Geometry: final body of the model. Coordinates: model frame, mm. Face numbers are marked on the shaded views. A direction names the side the tool comes from. Coordinates: 2 decimals unless noted, no trailing zeros. Write each loop counter-clockwise with the first axis right and the second up, starting at its lowest first coordinate (ties: lowest second). Pieces come first, ordered by that corner, then holes. Notation, with made-up numbers: M 68.25,5.5 L 87.25,5.5 A33 ccw 87.25,34.5 Z; hole C 78,62 d7. An arc over 180 degrees is marked long. Write item = value, one per line. Start each with the question number.
Item 1: First-contact query: pin 1 Ø10 at (x, z) = (-21.5, 1.5) entering from -Y; pin 2 Ø3 at (y, z) = (-2.5, -4) entering from +X; pin 3 Ø1.5 at (y, z) = (16.5, 2) entering from -X. Flat tips, straight axial feed; report the tip coordinate or a pass-through.
Item 2: Pull-direction query (X, two-part tool) for the marked faces 3, 4 and 5; classes: +X half, -X half, draft (parallel to the pull), parting line (faces both ways), or undercut.
Item 3: Section B-B on z = -39. Output: boundary loops of the cut face in (x, y).
Item 4: Section A-A on z = 25. Output: boundary loops of the cut face in (x, y).
Item 5: Reachability of the marked faces 1 and 2 from +Z, -Z, +X, -X, +Y, -Y: full face, straight path, thin tool, end or side. Return the list, or none.
Item 6: Ray query, L1, parallel to Y at x = 0, z = 20; L2, parallel to Z at x = -8.5, y = 2.5; L3, parallel to X at y = -14.5, z = 9.5. Return the intervals inside material, ascending. Write a range as [from, to].
Autodesk Inventor part; units mm, degrees
ref_plane "YZ Plane" through (0, 0, 0) normal (1, 0, 0) x (0, 1, 0)
ref_plane "XZ Plane" through (0, 0, 0) normal (0, 1, 0) x (-1, 0, 0)
ref_plane "XY Plane" through (0, 0, 0) normal (0, 0, 1) x (1, 0, 0)
sketch "スケッチ1" plane through (0, 0, 0) normal (0, 0, 1) x (1, 0, 0)
  circle A0 centre (0, 0) radius 30
  circle A1 centre (0, 0) radius 19.5
  dimension "d0" = 60
  dimension "d1" = 39
extrude "押し出し1" add sketch "スケッチ1" along normal blind 30
sketch "スケッチ3" plane through (0, 0, 0) normal (0, 0, -1) x (-1, 0, 0)
  circle A0 centre (0, 0) radius 30
  circle A1 centre (0, 0) radius 19.5
extrude "押し出し2" add sketch "スケッチ3" along normal blind 5 contours A0 | A1
sketch "スケッチ4" plane through (0, 0, -5) normal (0, 0, -1) x (-1, 0, 0)
  circle A0 centre (0, 0) radius 6
  dimension "d6" = 12
extrude "押し出し3" add sketch "スケッチ4" along normal blind 40
chamfer "面取り1" distance 10 angle 45 1 edges at (30, 0, -5)
properties part number "encoder_shaft_3D プリント"
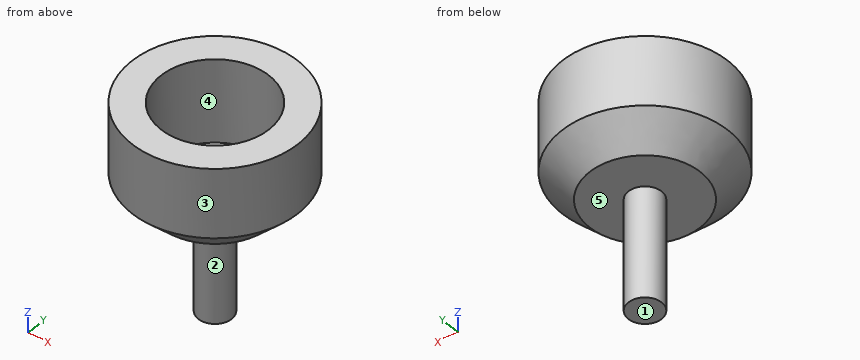
Responses:
q1.pin_1 = -24.05
q1.pin_2 = 22.37
q1.pin_3 = -22.46
q2.face_3 = parting line
q2.face_4 = undercut
q2.face_5 = draft
q3.outline = C 0,0 d12
q4.outline = C 0,0 d60; hole C 0,0 d39
q5.face_1 = -Z, +X, -X, +Y, -Y
q5.face_2 = -Z
q6.L1 = [-30, -19.5], [19.5, 30]
q6.L2 = [-5, 0]
q6.L3 = [-26.26, -13.04], [13.04, 26.26]
